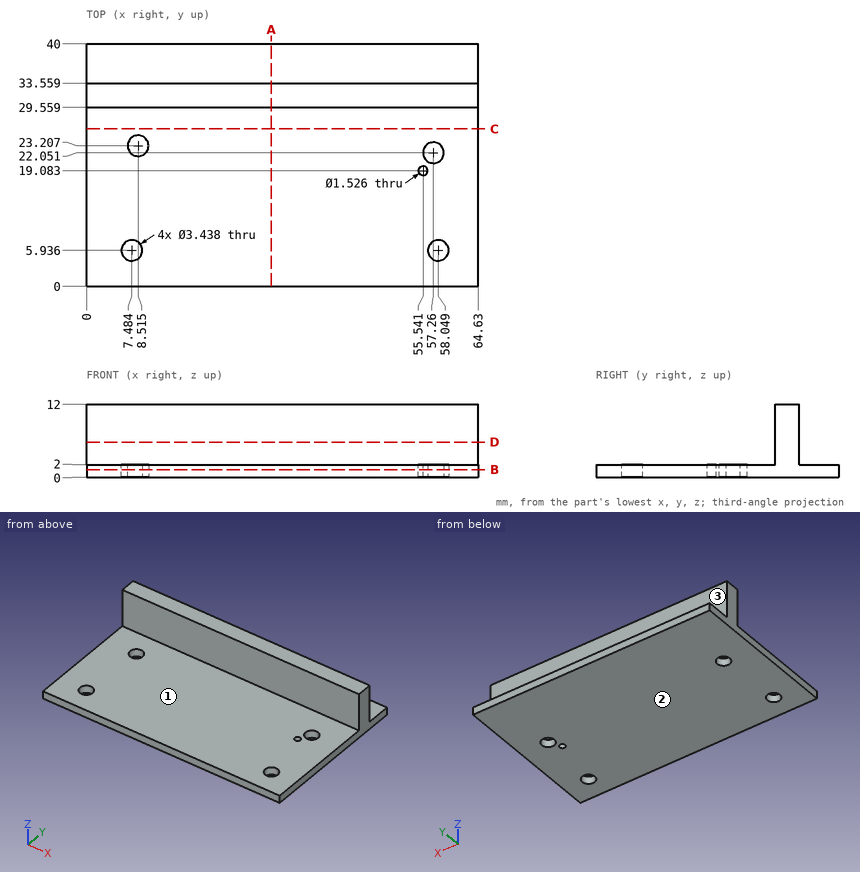
Answer from the drawing. Dimensions are ordinates in mm from the lowest x, y and z of the part. A direction names the side the tool comes from. Coordinates: 2 decimals unless noted, no trailing zeros. Loops run counter-clockwise (first coordinate to the right, second up) from the corner with the lowest first, then second, coordinate; pieces in that order, holes last. Notation, with made-up numbers: (51, 23) -> (88, 23) arc R38 ccw to (88, 61) -> close; hole circle Ø5 at (75, 10). An arc over 180 degrees is marked (long way). Return JSON: item names as keys, results as strings.
Item 1: Find section B-B (z = 1.25). Determine the outline of the cut face in (x, y) (1 decimal), plus the area to 3 significant figures.
Answers:
{"outline": "(0, 0) -> (64.6, 0) -> (64.6, 40) -> (0, 40) -> close; hole circle Ø3.4 at (7.5, 5.9); hole circle Ø3.4 at (8.5, 23.2); hole circle Ø1.5 at (55.5, 19.1); hole circle Ø3.4 at (57.3, 22.1); hole circle Ø3.4 at (58, 5.9)", "area": "2,550 mm2"}
Item 2: Flat-ended cylindrical pins translate along their axes: P1, Ø5.5, axis at x = 58.05, y = 5.94, coming from the +Z side; P2, Ø3, axis at x = 21.5, z = 8, coming from the -Y side. Find the tip coordinate at first contact, or state that the pin passes through.
Answers:
{"P1": "stops at z = 2", "P2": "stops at y = 29.56"}
Item 3: Find section D-D (z = 5.75). Determine the outline of the cut face in (x, y).
Answers:
{"outline": "(0, 29.56) -> (64.63, 29.56) -> (64.63, 33.56) -> (0, 33.56) -> close"}
Item 4: Find section A-A (x = 30.5). Determine the outline of the cut face in (y, z), plus the area to 3 significant figures.
Answers:
{"outline": "(0, 0) -> (40, 0) -> (40, 2) -> (33.56, 2) -> (33.56, 12) -> (29.56, 12) -> (29.56, 2) -> (0, 2) -> close", "area": "120 mm2"}
Item 5: Find the intervals of material crossed by probe 1 along X at (y, z) = (7, 1) (1 decimal); probe 2 along Y at (x, z) = (16.5, 5.75); probe 3 along Z at (x, y) = (19, 2), in increasing order.
Answers:
{"probe 1": "x = 0 to 6.1, 8.8 to 56.7, 59.4 to 64.6", "probe 2": "y = 29.56 to 33.56", "probe 3": "z = 0 to 2"}
Item 6: Find section C-C (y = 26). Determine the outline of the cut face in (x, z).
Answers:
{"outline": "(0, 0) -> (64.63, 0) -> (64.63, 2) -> (0, 2) -> close"}
Item 7: For the marked faces 1, 2 and 3, determine the directions among +Z, -Z, +X, -X, +Y, -Y from which every point of the face is accessible in a straight line to the end or side of a thin tool.
Answers:
{"face 1": "+Z, +X, -X, -Y", "face 2": "-Z, +X, -X, +Y, -Y", "face 3": "+Z, +X, -X, +Y"}
